For this review, take the finished solid that the model builds, in its own axes (mm). A direction names the side the tool comes from. Coordinates: 2 decimals unless noted, no trailing zeros. Loops run counter-clockwise (first coordinate to the right, second up) from the corner with the lowest first, then second, coordinate; pieces in that order, holes last.
```python
from build123d import *

# Parameters (mm, degrees)
F0_R     = 30
F1_DEPTH = 600
F3_DEPTH = 20
F4_R     = 17.5
F5_DEPTH = 50


with BuildPart() as f1:
    # F0 (on Top) → F1 (new body)
    with BuildSketch(Plane.XY):
        Circle(F0_R)
    extrude(amount=F1_DEPTH)

    # F2 (on Right) → F3 (join, symmetric)
    with BuildSketch(Plane.YZ):
        with BuildLine():
            Line((-29.826352, 0), (-34.819973, -49.043968))
            ThreePointArc((-34.819973, -49.043968), (-0.122433, -87.589098), (34.843925, -49.287659))
            Line((34.843925, -49.287659), (30.173648, 0))
            Line((30.173648, 0), (-29.826352, 0))
        make_face()
    extrude(amount=F3_DEPTH, both=True)

    # F4 (on face) → F5 (cut)
    with BuildSketch(Plane(origin=(-20, 0, 0), x_dir=(0, -1, 0), z_dir=(-1, 0, 0))):
        with Locations((0, -52.589312)):
            Circle(F4_R)
    extrude(amount=-F5_DEPTH, mode=Mode.SUBTRACT)


solid = f1.part
```
Q1. Wall thickness on probe 1 along Z at (x, y) = (-0.5, 0); probe 2 along Y at (x, z) = (0, 469); probe 3 along X at (y, z) = (1.5, 41): over which ranges is each line inside the solid? List them lowest first.
Q2. Machinability: for faces 1 (the face through (20, 0, -33)), 2 (the face through (0, 0, 600)), 3 (the face through (-29.97, 1.32, 295.8)), which of the approach directions +Z, -Z, +X, -X, +Y, -Y give a long, thin tool a straight path to every point of the face, cutting with its end or side? Answer none if there is none.
Q3. Consider section A-A (y = 0). State the section outline as (x, z) points, then the cut area to 3 significant figures.
Q4. For pin 1 Ø11 at (x, y) = (24.5, 8.5) entering from -Z; pin 2 Ø10 at (y, z) = (21.5, 497) entering from +X; pin 3 Ø4 at (x, z) = (8.5, 41.5) entering from +Y, all flat-tipped, find the tip position at first contact; note any pin that passes through.
Q5. Consider section C-C (z = 433.5). State the section outline as (x, y) points.
Q6. The part is to be moulded in two halves that separate along Z. For faces 4 (the face through (0.28, -32.29, -24.18)), 5 (the face through (-0.28, 3.794, -69.673)), 6 (the face through (-20, 0, -33)), say which applies: +Z half, -Z half, draft (parallel to the pull), parting line (faces both ways), or undercut.
Q7. Consider section B-B (x = -10). State the section outline as (y, z) points.
Model answer:
1. probe 1: z = -87.59 to -70.09, -35.09 to 600
1. probe 2: y = -30 to 30
1. probe 3: x = -29.96 to 29.96
2. face 1: -Z, +X, +Y, -Y
2. face 2: +Z, +X, -X, +Y, -Y
2. face 3: +Z
3. outline: (-30, 0) - (-20, 0) - (-20, -35.09) - (20, -35.09) - (20, 0) - (30, 0) - (30, 600) - (-30, 600) - close; (-20, -87.59) - (20, -87.59) - (20, -70.09) - (-20, -70.09) - close
3. area: 38,100 mm2
4. pin 1: stops at z = -87.18
4. pin 2: stops at x = 25.05
4. pin 3: stops at y = 29.29
5. outline: circle Ø60 at (0, 0)
6. face 4: +Z half
6. face 5: undercut
6. face 6: draft
7. outline: (-34.82, -49.04) arc R35 ccw (long way) to (34.84, -49.29) - (30.17, 0) - (28.28, 0) - (28.28, 600) - (-28.28, 600) - (-28.28, 0) - (-29.83, 0) - close; hole circle Ø35 at (0, -52.59)
